Check sheet for the modelled part. Datum: model origin and axes. Units: mm. Face numbers are marked on the shaded views. A direction names the side the tool comes from. Round coordinates to 2 decimals unless told otherwise and drop trailing zeros. Loops run counter-clockwise (first coordinate to the right, second up) from the corner with the lowest first, then second, coordinate; pieces in that order, holes last. Notation, with made-up numbers: (-18, 29) -> (31, 29) arc R18 ccw to (31, 44) -> close; hole circle Ø2 at (24, 45). An arc over 180 degrees is marked (long way). Return JSON: item names as keys, results as strings.
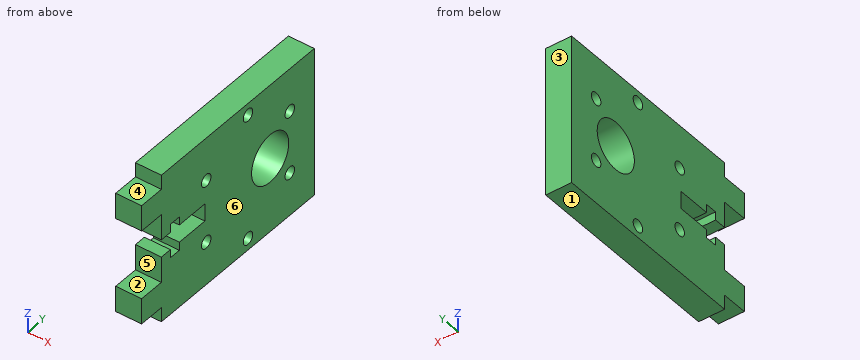
from build123d import *

# Parameters (mm, degrees)
MOTOR_PLATE_R       = 1.524
MOTOR_PLATE_R_2     = 5.969
BOSS_EXTRUDE1_DEPTH = 6.35


with BuildPart() as part:
    # Motor plate → Boss-Extrude1 (new body)
    with BuildSketch(Plane(origin=(0, 0, 0), x_dir=(0, 0, -1), z_dir=(1, 0, 0))):
        Polygon((-18.415, -24.552598803), (-14.859, -24.552598803), (-14.859, -30.902598803), (-8.509, -30.902598803), (-8.509, -24.552598803), (-2.159, -24.552598803), (-2.159, -21.684895821), (-4.199999982, -21.684895821), (-4.199999982, -18.784895779), (-2.159, -18.784895779), (-2.159, -10.582598803), (2.159, -10.582598803), (2.159, -18.784895779), (4.199999982, -18.784895779), (4.199999982, -21.684895821), (2.159, -21.684895821), (2.159, -24.552598803), (8.509, -24.552598803), (8.509, -30.902598803), (14.859, -30.902598803), (14.859, -24.552598803), (18.415, -24.552598803), (18.415, 24.552598803), (-18.415, 24.552598803), align=None)
        with Locations((7.747, 16.678598803)):
            Circle(MOTOR_PLATE_R, mode=Mode.SUBTRACT)
        with Locations((15.494, 3.260401197)):
            Circle(MOTOR_PLATE_R, mode=Mode.SUBTRACT)
        with Locations((7.747, -10.157796409)):
            Circle(MOTOR_PLATE_R, mode=Mode.SUBTRACT)
        with Locations((-7.747, -10.157796409)):
            Circle(MOTOR_PLATE_R, mode=Mode.SUBTRACT)
        with Locations((-15.494, 3.260401197)):
            Circle(MOTOR_PLATE_R, mode=Mode.SUBTRACT)
        with Locations((-7.747, 16.678598803)):
            Circle(MOTOR_PLATE_R, mode=Mode.SUBTRACT)
        with Locations((0, 10.372401197)):
            Circle(MOTOR_PLATE_R_2, mode=Mode.SUBTRACT)
    extrude(amount=BOSS_EXTRUDE1_DEPTH)


solid = part.part
Q1. Tool access check on the marked faces 5 and 6. Record the directions out of +Z, -Z, +X, -X, +Y, -Y that give a thin tool (end or side, any length) a straight path to the whole face; none if there is none.
Results list:
{"face 5": "+X, -X, -Y", "face 6": "+Z, -Z, +X, +Y, -Y"}
Q2. Section check A-A (z = 0). Record the boundary of the cut face in (x, y), then the cut area to 3 significant figures.
Results list:
{"outline": "(0, -10.58) -> (6.35, -10.58) -> (6.35, 4.4) -> (0, 4.4) -> close; (0, 16.34) -> (6.35, 16.34) -> (6.35, 24.55) -> (0, 24.55) -> close", "area": "147 mm^2"}
Q3. Draft check along Z on the marked faces 1, 2, 3 and 4. Enter one of: released by +Z, released by -Z, zero draft, split by the parting line, or undercut.
Results list:
{"face 1": "released by -Z", "face 2": "undercut", "face 3": "zero draft", "face 4": "released by +Z"}
Q4. Section check C-C (x = 4). Count the separate pieces of the cut face and the enclosed holes in it, then the cut area to 3 significant figures.
Results list:
{"separate pieces": "1", "enclosed holes": "7", "area": "1,660 mm^2"}
Q5. Go/stop test with flat-tipped pins: pin 1 (1 mm diameter, centred on x = 1, z = 0.5, fed in from -Y); pin 2 (3 mm diameter, centred on x = 4.5, y = -26.5, fed in from -Z); pin 3 (2 mm diameter, centred on x = 2, z = 3.5, fed in from -Y). Record where each tip stops, or that it passes through.
Results list:
{"pin 1": "y = -10.58", "pin 2": "z = -14.86", "pin 3": "y = -24.55"}
Q6. Section check B-B (y = -21). Record the boundary of the cut face in (x, z) (3 decimals).
Results list:
{"outline": "(0, -18.415) -> (6.35, -18.415) -> (6.35, -4.2) -> (0, -4.2) -> close; (0, 4.2) -> (6.35, 4.2) -> (6.35, 18.415) -> (0, 18.415) -> close"}
Q7. Section check D-D (z = 7.5). Record the boundary of the cut face in (x, y).
Results list:
{"outline": "(0, -24.55) -> (6.35, -24.55) -> (6.35, -11.66) -> (0, -11.66) -> close; (0, -8.65) -> (6.35, -8.65) -> (6.35, 15.17) -> (0, 15.17) -> close; (0, 18.18) -> (6.35, 18.18) -> (6.35, 24.55) -> (0, 24.55) -> close"}
Q8. Material ranges on line 1 (Z direction, x = 3.25, y = -23) (3 decimals); line 2 (Z direction, x = 3.75, y = -27.5); line 3 (Y direction, x = 2.75, z = -16), recorded low to high.
Results list:
{"line 1": "-18.415 to -2.159, 2.159 to 18.415", "line 2": "-14.86 to -8.51, 8.51 to 14.86", "line 3": "-24.55 to 1.82, 4.7 to 24.55"}
